```python
from build123d import *

# Parameters (mm, degrees)
SKIZZE1_W                       = 42
SKIZZE1_H                       = 42
SKIZZE1_R                       = 12
SKIZZE1_R_2                     = 2.5
AUFSATZ_LINEAR_AUSTRAGEN1_DEPTH = 10
SKIZZE2_R                       = 1
SCHNITT_LINEAR_AUSTRAGEN1_DEPTH = 8
M4_GEWINDEBOHRUNG1_D            = 3.3
M4_GEWINDEBOHRUNG1_DEPTH        = 11.5
M4_GEWINDEBOHRUNG1_CSINK_D      = 4.05
M4_GEWINDEBOHRUNG1_CSINK_ANGLE  = 90
M4_GEWINDEBOHRUNG1_TIP          = 0.991420021


with BuildPart() as part:
    # Skizze1 → Aufsatz-Linear austragen1 (new body)
    with BuildSketch(Plane.XY):
        with Locations((-7.301275723, -4.674228082)):
            Rectangle(SKIZZE1_W, SKIZZE1_H)
        with Locations((-7.301275723, -4.674228082)):
            Circle(SKIZZE1_R, mode=Mode.SUBTRACT)
        with Locations((-22.801275723, 10.825771918)):
            Circle(SKIZZE1_R_2, mode=Mode.SUBTRACT)
        with Locations((8.198724277, 10.825771918)):
            Circle(SKIZZE1_R_2, mode=Mode.SUBTRACT)
        with Locations((-22.801275723, -20.174228082)):
            Circle(SKIZZE1_R_2, mode=Mode.SUBTRACT)
        with Locations((8.198724277, -20.174228082)):
            Circle(SKIZZE1_R_2, mode=Mode.SUBTRACT)
    extrude(amount=AUFSATZ_LINEAR_AUSTRAGEN1_DEPTH)

    # Skizze2 → Schnitt-Linear austragen1 (cut)
    with BuildSketch(Plane.ZY.offset(28.301275723)):
        with Locations((4, 4.325771918)):
            Circle(SKIZZE2_R)
        with Locations((4, -13.674228082)):
            Circle(SKIZZE2_R)
    extrude(amount=-SCHNITT_LINEAR_AUSTRAGEN1_DEPTH, mode=Mode.SUBTRACT)

    # M4 Gewindebohrung1
    with Locations(Plane(origin=(-28.301275723, 4.325771918, 4), x_dir=(0, 0, -1), z_dir=(-1, 0, 0))):
        with Locations((0, 0), (0, 18)):
            CounterSinkHole(M4_GEWINDEBOHRUNG1_D / 2, M4_GEWINDEBOHRUNG1_CSINK_D / 2, depth=M4_GEWINDEBOHRUNG1_DEPTH, counter_sink_angle=M4_GEWINDEBOHRUNG1_CSINK_ANGLE)
            with Locations((0, 0, -(M4_GEWINDEBOHRUNG1_DEPTH + M4_GEWINDEBOHRUNG1_TIP / 2))):  # 118° drill point
                Cone(0, M4_GEWINDEBOHRUNG1_D / 2, M4_GEWINDEBOHRUNG1_TIP, mode=Mode.SUBTRACT)


solid = part.part
```
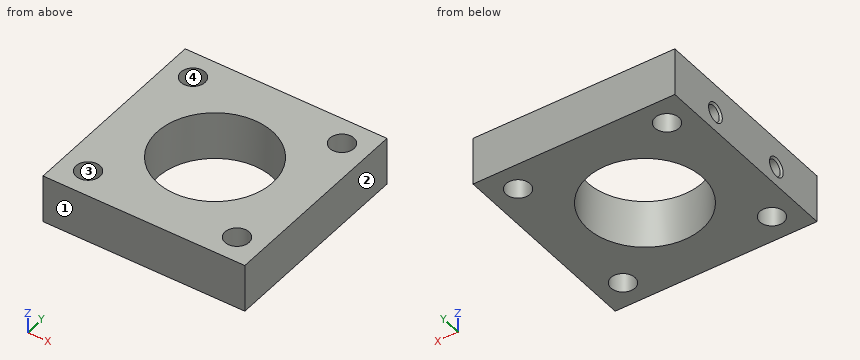
The listing builds one solid part. Answer for the finished solid, in the listing's coordinates (mm). Face numbers are marked on the shaded views. Coordinates: 2 decimals unless noted, no trailing zeros. Loops run counter-clockwise (first coordinate to the right, second up) from the corner with the lowest first, then second, coordinate; pieces in that order, holes last. Notation, with made-up numbers: (41.5, 41.5) - (87.5, 41.5) arc R25 ccw to (87.5, 67.5) - close; hole circle Ø10 at (75, 16.25). An arc over 180 degrees is marked (long way). Use a Markdown table: item, result. Add a question column.
1) The part is cut by section A-A, the plane x = -14.5. Give the vertices of the cut face in (y, z).
2) The part is cut by section C-C, the plane z = 8. Give the vertices of the cut face in (x, y).
3) The part is cut by section D-D, the plane x = 9. Give the vertices of the cut face in (y, z).
4) The mould has two halves that part along X. Classify the marked faces 1, 2, 3 and 4: released by +X, released by -X, zero draft, split by the parting line, or undercut.
5) Given pin 1 (2.5 mm diameter, centred on y = -13.67, z = 4, fed in from -X), flat-ended and moving along its own axis, determine where the tip first touches the part or whether it passes through.
6) Find the intervals of material crossed by line 1 (Y direction, x = 7, z = 4.75); line 2 (Y direction, x = -25.5, z = 4.25); line 3 (X direction, y = 11.5, z = 9.5), in increasing order.
7) The part is cut by section B-B, the plane y = 1.5. Give the vertices of the cut face in (x, z).
Here are the results:
| question | item | result |
|---|---|---|
| 1 | outline | (-25.67, 0) - (-14.28, 0) - (-14.28, 10) - (-25.67, 10) - close; (4.93, 0) - (16.33, 0) - (16.33, 10) - (4.93, 10) - close |
| 2 | outline | (-28.3, -25.67) - (13.7, -25.67) - (13.7, 16.33) - (-28.3, 16.33) - close; hole circle Ø5 at (-22.8, -20.17); hole circle Ø5 at (-22.8, 10.83); hole circle Ø24 at (-7.3, -4.67); hole circle Ø5 at (8.2, -20.17); hole circle Ø5 at (8.2, 10.83) |
| 3 | outline | (-25.67, 0) - (-22.54, 0) - (-22.54, 10) - (-25.67, 10) - close; (-17.81, 0) - (8.46, 0) - (8.46, 10) - (-17.81, 10) - close; (13.19, 0) - (16.33, 0) - (16.33, 10) - (13.19, 10) - close |
| 4 | face 1 | zero draft |
| 4 | face 2 | released by +X |
| 4 | face 3 | undercut |
| 4 | face 4 | undercut |
| 5 | pin 1 | stops at x = -16.56 |
| 6 | line 1 | y = -25.67 to -22.37, -17.98 to 8.63, 13.02 to 16.33 |
| 6 | line 2 | y = -25.67 to -15.31, -12.04 to 2.69, 5.96 to 16.33 |
| 6 | line 3 | x = -28.3 to -25.21, -20.39 to 5.79, 10.61 to 13.7 |
| 7 | outline | (-28.3, 0) - (-17.59, 0) - (-17.59, 10) - (-28.3, 10) - close; (2.99, 0) - (13.7, 0) - (13.7, 10) - (2.99, 10) - close |
